```python
from build123d import *

# Parameters (mm, degrees)
SKETCH1_R           = 14
BOSS_EXTRUDE1_DEPTH = 175
SKETCH5_W           = 7
SKETCH5_H           = 23.880326309


with BuildPart() as part:
    # Sketch1 → Boss-Extrude1 (new body)
    with BuildSketch(Plane(origin=(0, 0, 0), x_dir=(0, 0, -1), z_dir=(1, 0, 0))):
        with BuildLine():
            ThreePointArc((-14, 19.49358869), (-24, 0), (-14, -19.49358869))
            ThreePointArc((-14, -19.49358869), (-11.620285492, -25.23872773), (-14, -30.98386677))
            ThreePointArc((-14, -30.98386677), (0, -34), (14, -30.98386677))
            ThreePointArc((14, -30.98386677), (11.620285492, -25.23872773), (14, -19.49358869))
            ThreePointArc((14, -19.49358869), (24, 0), (14, 19.49358869))
            ThreePointArc((14, 19.49358869), (11.620285492, 25.23872773), (14, 30.98386677))
            ThreePointArc((14, 30.98386677), (-0.111150927, 33.999818315), (-14.202281174, 30.891668933))
            ThreePointArc((-14.202281174, 30.891668933), (-11.740520876, 25.234522614), (-14, 19.49358869))
        make_face()
        Circle(SKETCH1_R, mode=Mode.SUBTRACT)
    extrude(amount=BOSS_EXTRUDE1_DEPTH)

    # Sketch5 → Cut-Revolve1 (revolve, cut)
    with BuildSketch(Plane.XY, mode=Mode.PRIVATE) as cut_revolve1_sk:
        with Locations((151.5, 29.440163155)):
            Rectangle(SKETCH5_W, SKETCH5_H)
    revolve(cut_revolve1_sk.sketch.rotate(Axis((175, 0, 0), (-1, 0, 0)), 90), axis=Axis((175, 0, 0), (-1, 0, 0)), mode=Mode.SUBTRACT)


solid = part.part
```
Could you check a few things on this model? Use its own coordinates, in mm. A direction names the side the tool comes from. Round coordinates to 2 decimals unless told otherwise and drop trailing zeros. Loops run counter-clockwise (first coordinate to the right, second up) from the corner with the lowest first, then second, coordinate; pieces in that order, holes last. Notation, with made-up numbers: (-6, 4.25) - (8, 4.25) arc R25 cw to (8, 27.25) - close; hole circle Ø2 at (68.25, 85.5). An arc over 180 degrees is marked (long way). Use CSV: the item, a comma, the result in double quotes.
Item 1: I need wall thicknesses on L1, parallel to Y at x = 89, z = 0; L2, parallel to X at y = -29, z = -5.5; L3, parallel to Z at x = 105, y = 0.5. Which ranges of each line are inside material? Lowest first, please. Write a range as [from, to].
Here are the results:
L1,"y = [-34, -14], [14, 34]"
L2,"x = [0, 148], [155, 175]"
L3,"z = [-23.99, -13.99], [13.99, 23.99]"
Item 2: If we section it at D-D on x = 153: List the corners of the cut face in (y, z) for me, then the cut area to 3 significant figures.
Here are the results:
outline,"circle Ø35 at (0, 0); hole circle Ø28 at (0, 0)"
area,"346 mm²"
Item 3: If we section it at C-C on y = 0: List the corners of the cut face in (x, z) for me.
Here are the results:
outline,"(0, -24) - (148, -24) - (148, -17.5) - (155, -17.5) - (155, -24) - (175, -24) - (175, -14) - (0, -14) - close; (0, 14) - (175, 14) - (175, 24) - (155, 24) - (155, 17.5) - (148, 17.5) - (148, 24) - (0, 24) - close"
Item 4: If we mould it in two halves opening along X, with no side actions, what happens to faces 3 (the cylindrical face through (72.96, 25.15, -11.62)), 4 (the flat face through (175, -15, 0)), 5 (the cylindrical face through (151.549, 17.084, 3.794))? For each: pulls with the +X half, pulls with the -X half, needs draft (parallel to the pull), parting line crosses it, or undercut.
Here are the results:
face 3,"needs draft"
face 4,"pulls with the +X half"
face 5,"undercut"
Item 5: If we section it at A-A on z = 0: List the corners of the cut face in (x, y) for me.
Here are the results:
outline,"(0, -34) - (148, -34) - (148, -17.5) - (155, -17.5) - (155, -34) - (175, -34) - (175, -14) - (0, -14) - close; (0, 14) - (175, 14) - (175, 34) - (155, 34) - (155, 17.5) - (148, 17.5) - (148, 34) - (0, 34) - close"
Item 6: Will these pins go through, and if not, where does the flat tip stop? pin 1 (3 mm diameter, centred on x = 110, z = 2, fed in from -Y); pin 2 (1 mm diameter, centred on x = 156.5, z = -15, fed in from +Y); pin 3 (10 mm diameter, centred on x = 59, z = -11.5, fed in from +Y); pin 4 (22.5 mm diameter, centred on y = 0, z = 0, fed in from -X).
Here are the results:
pin 1,"stops at y = -34"
pin 2,"stops at y = 19.12"
pin 3,"stops at y = 33.37"
pin 4,"passes through"
Item 7: For faces 1 (the cylindrical face through (72.96, -25.15, 11.62)), 2 (the flat face through (155, -8, -16)), which set-ups out of +Z, -Z, +X, -X, +Y, -Y let a thin tool reach every point of the face, with its end or its side?
Here are the results:
face 1,"+Z, +X, -X"
face 2,"none"
Item 8: If we section it at B-B on x = 122: List the corners of the cut face in (y, z) for me.
Here are the results:
outline,"(-30.98, -14) arc R8.12 cw to (-19.49, -14) arc R24 ccw to (19.49, -14) arc R8.12 cw to (30.98, -14) arc R34 ccw to (30.89, 14.2) arc R8.06 cw to (19.49, 14) arc R24 ccw to (-19.49, 14) arc R8.12 cw to (-30.98, 14) arc R34 ccw to start; hole circle Ø28 at (0, 0)"
